Autodesk Inventor part; units mm, degrees
ref_plane "Deaktiviert_NICHT_mehrverwenden_Zyl__Schraube_DIN_EN_ISO_4762_XY" through (0, 0, 0) normal (0, 1, 0) x (1, 0, 0)
ref_plane "Deaktiviert_NICHT_mehrverwenden_Zyl__Schraube_DIN_EN_ISO_4762_YZ" through (0, 0, 0) normal (1, 0, 0) x (0, 0, -1)
ref_plane "Deaktiviert_NICHT_mehrverwenden_Zyl__Schraube_DIN_EN_ISO_4762_ZX" through (0, 0, 0) normal (0, 0, -1) x (0, 1, 0)
sketch "Skizze_1" plane through (0, 0, 0) normal (0, 0, 1) x (1, 0, 0)
  line L0 (0, -30) -> (0, 0)
  line L1 (0, 0) -> (3, 0)
  line L2 (3, 0) -> (3, -29.3865)
  line L3 (3, -29.3865) -> (2.3865, -30)
  line L4 (2.3865, -30) -> (0, -30)
  line L5 (0, -30) -> (0, 0)
revolve "Revolution1" add sketch "Skizze_1" angle 360 about axis through (0, -30, 0) along (0, -1, 0)
thread "Thread1"
sketch "Skizze_2" plane through (0, 0, 0) normal (0, 0, 1) x (1, 0, 0)
  line L0 (0, 0) -> (0, 4)
  line L1 (0, 4) -> (4.5, 4)
  arc A0 (5, 3.5) -> (4.5, 4) centre (4.5, 3.5) ccw
  line L2 (5, 3.5) -> (5, 0)
  line L3 (5, 0) -> (0, 0)
  line L4 (0, 0) -> (0, 4)
revolve "Revolution2" add sketch "Skizze_2" angle 360 about axis through (0, 0, 0) along (0, -1, 0)
sketch "Skizze_3" plane through (0, 4, 0) normal (0, 1, 0) x (1, 0, 0)
  line L0 (-2, -1.1547) -> (0, -2.3094)
  line L1 (0, -2.3094) -> (2, -1.1547)
  line L2 (2, -1.1547) -> (2, 1.1547)
  line L3 (2, 1.1547) -> (0, 2.3094)
  line L4 (0, 2.3094) -> (-2, 1.1547)
  line L5 (-2, 1.1547) -> (-2, -1.1547)
extrude "Extrusion1" cut sketch "Skizze_3" against normal blind 4
ref_plane "EP_XY" through (0, 0, 0) normal (0, 1, 0) x (1, 0, 0)
ref_plane "EP_YZ" through (0, 0, 0) normal (1, 0, 0) x (0, 0, -1)
ref_plane "EP_ZX" through (0, 0, 0) normal (0, 0, -1) x (0, 1, 0)
ref_plane "EP_Schraube_XY" through (0, 0, 0) normal (0, 1, 0) x (1, 0, 0)
ref_plane "EP_Schraube_YZ" through (0, 0, 0) normal (1, 0, 0) x (0, 0, -1)
ref_plane "EP_Schraube_ZX" through (0, 0, 0) normal (0, 0, -1) x (0, 1, 0)
properties part number "Zyl.Schr-M6x30_Stahl_X094085"
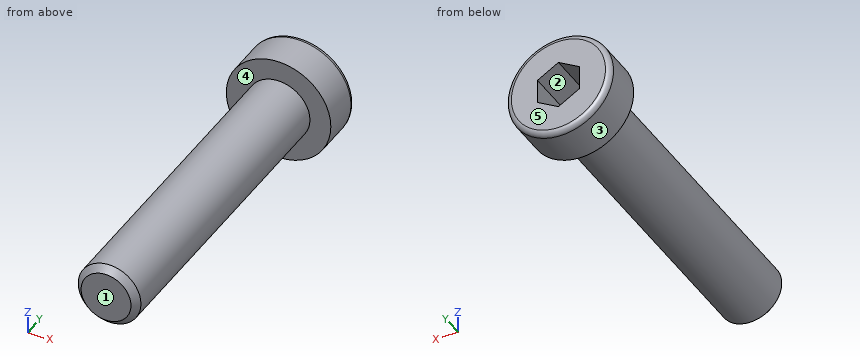
Geometry: final body of the model. Coordinates: model frame, mm. Face numbers are marked on the shaded views. A direction names the side the tool comes from. Round coordinates to 2 decimals unless told otherwise and drop trailing zeros. Loops run counter-clockwise (first coordinate to the right, second up) from the corner with the lowest first, then second, coordinate; pieces in that order, holes last.
Q1. Material intervals for L1, parallel to Y at x = -0.75, z = 1.5; L2, parallel to Y at x = 2.25, z = -3.75; L3, parallel to Z at x = 1, y = 2, sorted ascending.
Q2. Pin query (flat end, axial travel): P1, Ø2, axis at x = -0.5, z = 0, coming from the +Y side; P2, Ø3, axis at x = -2, y = -21, coming from the +Z side; P3, Ø3, axis at x = 3, y = -20, coming from the -Z side. Return the tip coordinate at first contact, or that it passes through.
Q3. Section A-A on y = 1. Return loops of the section in (x, z).
Q4. Pull-direction query (X, two-part tool) for the marked faces 1, 2 and 3; classes: released by +X, released by -X, zero draft, split by the parting line, or undercut.
Q5. Section B-B on z = 0. Return loops of the section in (x, y), plus the area to 3 significant figures.
Q6. Section C-C on y = -2.5. Return loops of the section in (x, z), plus the area to 3 significant figures.
Q7. Access query for the marked faces 4 and 5. Directions: +Z, -Z, +X, -X, +Y, -Y. A direction counts if a zero-diameter tool reaches every point of the face in a straight line with its end or side. Return the directions, or none.
Evaluation:
1. L1: y = -30 to 0
1. L2: y = 0 to 4
1. L3: z = -4.9 to -1.73, 1.73 to 4.9
2. P1: stops at y = 0
2. P2: stops at z = 2.96
2. P3: stops at z = -2.6
3. outline: circle Ø10 at (0, 0); hole (-2, -1.15) - (0, -2.31) - (2, -1.15) - (2, 1.15) - (0, 2.31) - (-2, 1.15) - close
4. face 1: zero draft
4. face 2: undercut
4. face 3: split by the parting line
5. outline: (-5, 0) - (-3, 0) - (-3, -29.39) - (-2.39, -30) - (2.39, -30) - (3, -29.39) - (3, 0) - (5, 0) - (5, 3.5) arc R0.5 ccw to (4.5, 4) - (2, 4) - (2, 0) - (-2, 0) - (-2, 4) - (-4.5, 4) arc R0.5 ccw to (-5, 3.5) - close
5. area: 204 mm2
6. outline: circle Ø6 at (0, 0)
6. area: 28.3 mm2
7. face 4: -Y
7. face 5: +Z, -Z, +X, -X, +Y
